Read the model definition and answer for the solid it produces. Units are mm, in the model's axes. A direction names the side the tool comes from. Round coordinates to 2 decimals unless told otherwise and drop trailing zeros. Write each loop counter-clockwise with the first axis right and the second up, starting at its lowest first coordinate (ties: lowest second). Pieces come first, ordered by that corner, then holes. Notation, with made-up numbers: (-11.75, -9) -> (31.25, -9) arc R15 cw to (31.25, 7) -> close; hole circle Ø6 at (-28, 54.25). An arc over 180 degrees is marked (long way). Return JSON: item names as keys, results as strings. Group by question number.
(1) A cutting plane is placed at A-A on x = -9. Give the vertices of the cut face in (y, z), then the cut area to 3 significant figures.
(2) Given pin 1 (1.5 mm diameter, centred on y = 113.5, z = 1.5, fed in from -X); pin 2 (1 mm diameter, centred on x = 91.5, z = 1.5, fed in from +Y); pin 3 (1.5 mm diameter, centred on x = 22.5, z = 1.5, fed in from -Y), each flat-ended and moving along its own axis, determine where each tip first touches the part or whether it passes through.
(3) A cutting plane is placed at D-D on y = 14. Give the vertices of the cut face in (x, z), then the cut area to 3 significant figures.
(4) A cutting plane is placed at B-B on z = 1.8. State how many separate pieces and enclosed holes the cut face has, then the cut area to 3 significant figures.
(5) For faces 5 (the flat face through (-92.386, -59.982, 2.535)), 6 (the cylindrical face through (-99.41, 58.77, 2.54)), determine the directions among +Z, -Z, +X, -X, +Y, -Y from which every point of the face is accessible in a straight line to the end or side of a thin tool.
(6) A cutting plane is placed at C-C on y = 98. Give the vertices of the cut face in (x, z), then the cut area to 3 significant figures.
(7) The mould has two halves that part along Y. Classify faces 1 (the flat face through (-2, -20, 5)), 2 (the flat face through (58.705, -27.719, 2.535)), 3 (the flat face through (107.45, -63.89, 2.46)), 4 (the flat face through (87.17, 49.02, 2.46)): released by +Y, released by -Y, zero draft, split by the parting line, or undercut.
(8) Straight lines are drawn through the part: line 1 (Y direction, x = 27, z = 3.2); line 2 (Y direction, x = 62, z = 4); line 3 (Y direction, x = -88.5, z = 4.45). For each, find the intervals that lie inside material, in ascending order.
```python
from build123d import *

# Parameters (mm, degrees)
BOSS_EXTRUDE1_DEPTH = 5
BOSS_EXTRUDE2_DEPTH = 5
SKETCH4_W           = 10
SKETCH4_H           = 5
SKETCH4_W_2         = 29
CUT_EXTRUDE2_DEPTH  = 5
BOSS_EXTRUDE3_DEPTH = 5
SKETCH7_R           = 1.25
CUT_EXTRUDE4_DEPTH  = 5
FILLET2_R           = 10


with BuildPart() as part:
    # Sketch1 → Boss-Extrude1 (new body)
    with BuildSketch(Plane(origin=(0, 0, 0), x_dir=(0.8660254037844434, -0.49999999999999206, 0), z_dir=(0, 0, 1))):
        Polygon((125, -43.301270189), (125, 43.301270189), (-25, 129.903810568), (-100, 86.602540378), (-100, -86.602540378), (-25, -129.903810568), align=None)
    extrude(amount=BOSS_EXTRUDE1_DEPTH)

    # Sketch3 → Boss-Extrude2 (add)
    with BuildSketch(Plane.XY.offset(5)):
        Polygon((-86.602540378, -100), (86.602540378, -100), (129.903810568, -25), (43.301270189, 125), (-43.301270189, 125), (-129.903810568, -25), align=None)
    extrude(amount=-BOSS_EXTRUDE2_DEPTH)

    # Sketch4 → Cut-Extrude2 (cut)
    with BuildSketch(Plane.XY.offset(5)):
        with Locations((-35.05, 112.5)):
            Rectangle(SKETCH4_W, SKETCH4_H)
        with Locations((23.95, 112.5)):
            Rectangle(SKETCH4_W, SKETCH4_H)
        with Locations((-5.55, 112.5)):
            Rectangle(SKETCH4_W_2, SKETCH4_H)
        with Locations((-35.05, 62.1999492)):
            Rectangle(SKETCH4_W, SKETCH4_H)
        with Locations((23.95, 62.1999492)):
            Rectangle(SKETCH4_W, SKETCH4_H)
        with Locations((-5.55, 62.1999492)):
            Rectangle(SKETCH4_W_2, SKETCH4_H)
        Polygon((115.287794416, -20.315682578), (110.287794416, -28.975936616), (114.617921435, -31.475936616), (119.617921435, -22.815682578), align=None)
        Polygon((80.787794416, -80.07143544), (85.117921435, -82.57143544), (90.117921435, -73.911181402), (85.787794416, -71.411181402), align=None)
        Polygon((109.617921435, -40.136190654), (105.287794416, -37.636190654), (90.787794416, -62.750927364), (95.117921435, -65.250927364), align=None)
        Polygon((71.726672612, 4.834342822), (66.726672612, -3.825911216), (71.056799631, -6.325911216), (76.056799631, 2.334342822), align=None)
        Polygon((37.226672612, -54.92141004), (41.556799631, -57.42141004), (46.556799631, -48.761156002), (42.226672612, -46.261156002), align=None)
        Polygon((66.056799631, -14.986165254), (61.726672612, -12.486165254), (47.226672612, -37.600901964), (51.556799631, -40.100901964), align=None)
        Polygon((-75.237794416, -89.684317422), (-80.237794416, -81.024063384), (-84.567921435, -83.524063384), (-79.567921435, -92.184317422), align=None)
        Polygon((-109.737794416, -29.92856456), (-114.067921435, -32.42856456), (-109.067921435, -41.088818598), (-104.737794416, -38.588818598), align=None)
        Polygon((-89.567921435, -74.863809346), (-85.237794416, -72.363809346), (-99.737794416, -47.249072636), (-104.067921435, -49.749072636), align=None)
        Polygon((-31.676672612, -64.534292022), (-36.676672612, -55.874037984), (-41.006799631, -58.374037984), (-36.006799631, -67.034292022), align=None)
        Polygon((-66.176672612, -4.77853916), (-70.506799631, -7.27853916), (-65.506799631, -15.938793198), (-61.176672612, -13.438793198), align=None)
        Polygon((-46.006799631, -49.713783946), (-41.676672612, -47.213783946), (-56.176672612, -22.099047236), (-60.506799631, -24.599047236), align=None)
    extrude(amount=-CUT_EXTRUDE2_DEPTH, mode=Mode.SUBTRACT)

    # Sketch5 → Boss-Extrude3 (add)
    with BuildSketch(Plane.XY.offset(5)):
        with BuildLine():
            ThreePointArc((-43.301270189, 125), (-100.007931209, 57.739606004), (-129.903810568, -25))
            Line((-129.903810568, -25), (-43.301270189, 125))
        make_face()
        with BuildLine():
            ThreePointArc((-86.602540378, -100), (0, -115.479212009), (86.602540378, -100))
            Line((86.602540378, -100), (-86.602540378, -100))
        make_face()
    extrude(amount=-BOSS_EXTRUDE3_DEPTH)

    # Sketch7 → Cut-Extrude4 (cut)
    with BuildSketch(Plane.XY.offset(5)):
        with Locations((-99.474904421, 42.045588536)):
            Circle(SKETCH7_R)
        with Locations((34.707071641, 119.515588536)):
            Circle(SKETCH7_R)
        with Locations((113.447071641, -16.866092052)):
            Circle(SKETCH7_R)
        with Locations((-0.937563691, -82.906092052)):
            Circle(SKETCH7_R)
    extrude(amount=-CUT_EXTRUDE4_DEPTH, mode=Mode.SUBTRACT)

    # Fillet2
    fillet2_edges = [part.edges().sort_by_distance(p)[0] for p in [
        (-86.602540378, -100, 2.5),
        (-129.903810568, -25, 2.5),
        (-43.301270189, 125, 2.5),
        (43.301270189, 125, 2.5),
        (129.903810568, -25, 2.5),
        (86.602540378, -100, 2.5),
    ]]
    fillet(fillet2_edges, radius=FILLET2_R)


solid = part.part
```
Checks:
{
 "1": {"outline": "(-115.32, 0) -> (59.7, 0) -> (59.7, 5) -> (-115.32, 5) -> close; (64.7, 0) -> (110, 0) -> (110, 5) -> (64.7, 5) -> close; (115, 0) -> (125, 0) -> (125, 5) -> (115, 5) -> close", "area": "1,150 mm^2"},
 "2": {"pin 1": "stops at x = -56.98", "pin 2": "stops at y = 42.38", "pin 3": "stops at y = -114.53"},
 "3": {"outline": "(-119.93, 0) -> (107.39, 0) -> (107.39, 5) -> (-119.93, 5) -> close", "area": "1,140 mm^2"},
 "4": {"separate pieces": "1", "enclosed holes": "22", "area": "44,300 mm^2"},
 "5": {"face 5": "+Z, -Z", "face 6": "+Z, -Z, -X, +Y"},
 "6": {"outline": "(-71.09, 0) -> (58.89, 0) -> (58.89, 5) -> (-71.09, 5) -> close", "area": "650 mm^2"},
 "7": {"face 1": "zero draft", "face 2": "undercut", "face 3": "released by -Y", "face 4": "released by +Y"},
 "8": {"line 1": "y = -114.02 to 59.7, 64.7 to 110, 115 to 125", "line 2": "y = -107.67 to -22.01, -12.64 to 92.61", "line 3": "y = -96.71 to -74.25, -66.71 to 75.83"}
}
